```python
from build123d import *

# Parameters (mm, degrees)
PAD_DEPTH       = 5
SKETCH001_R     = 1.5
POCKET_DEPTH    = 2.751
SKETCH002_R     = 1
POCKET001_DEPTH = 5


with BuildPart() as part:
    # Sketch → Pad (new body, symmetric)
    with BuildSketch(Plane.YZ):
        with BuildLine():
            ThreePointArc((-1.299038, -0.75), (1.5, 0), (-1.299038, 0.75))
            Line((-11.299038, 0.75), (-1.299038, 0.75))
            Line((-11.299038, 2.75), (-11.299038, 0.75))
            Line((0, 2.75), (-11.299038, 2.75))
            ThreePointArc((1.2e-05, -2.75), (2.75, 6e-06), (0, 2.75))
            Line((-11.299038, -2.75), (1.2e-05, -2.75))
            Line((-11.299038, -2.75), (-11.299038, -0.75))
            Line((-11.299038, -0.75), (-1.299038, -0.75))
        make_face()
    extrude(amount=PAD_DEPTH, both=True)

    # Sketch001 → Pocket (cut, through all)
    with BuildSketch(Plane.XY):
        with Locations((0, -6)):
            Circle(SKETCH001_R)
    extrude(amount=-POCKET_DEPTH, mode=Mode.SUBTRACT)

    # Sketch002 → Pocket001 (cut)
    with BuildSketch(Plane.XY):
        with Locations((0, -6)):
            Circle(SKETCH002_R)
    extrude(amount=POCKET001_DEPTH, mode=Mode.SUBTRACT)


solid = part.part
```
The model under review builds one solid part; all positions refer to its coordinate system, in mm. A direction names the side the tool comes from. Round coordinates to 2 decimals unless told otherwise and drop trailing zeros. Loops run counter-clockwise (first coordinate to the right, second up) from the corner with the lowest first, then second, coordinate; pieces in that order, holes last.
1) Tool access review of faces 1 (the face through (-0.325, -7.464, -1.736)), 2 (the face through (-1, -7.5, -0.75)), 3 (the face through (1.2, -5.6, 2.75)): name each direction out of +Z, -Z, +X, -X, +Y, -Y from which nothing blocks a thin tool from reaching the whole face with its end or side.
Values follow:
face 1: -Z
face 2: +X, -X, -Y
face 3: +Z, +X, -X, +Y, -Y
2) Consider section D-D on x = 4.25. State the section outline as (y, z) points, then the cut area to 3 significant figures.
Values follow:
outline: (-11.3, -2.75) - (0, -2.75) arc R2.75 ccw to (0, 2.75) - (-11.3, 2.75) - (-11.3, 0.75) - (-1.3, 0.75) arc R1.5 cw (long way) to (-1.3, -0.75) - (-11.3, -0.75) - close
area: 52.2 mm2
3) Consider section B-B on y = -6. State the section outline as (x, z) points.
Values follow:
outline: (-5, -2.75) - (-1.5, -2.75) - (-1.5, -0.75) - (-5, -0.75) - close; (-5, 0.75) - (-1, 0.75) - (-1, 2.75) - (-5, 2.75) - close; (1, 0.75) - (5, 0.75) - (5, 2.75) - (1, 2.75) - close; (1.5, -2.75) - (5, -2.75) - (5, -0.75) - (1.5, -0.75) - close
4) Clearance check with a flat-ended pin moving along its axis: P1, Ø3, axis at x = -1, z = -2, coming from the +Y side. State where the tip first meets the part, or that it passes through.
Values follow:
P1: stops at y = 2.7
5) Consider section C-C on y = -1.75. State the section outline as (x, z) points, then the cut area to 3 significant figures.
Values follow:
outline: (-5, -2.75) - (5, -2.75) - (5, -0.75) - (-5, -0.75) - close; (-5, 0.75) - (5, 0.75) - (5, 2.75) - (-5, 2.75) - close
area: 40.0 mm2
6) The part is to be moulded in two halves that separate along Z. For faces 4 (the face through (0, -11.299, 2)), 5 (the face through (0.1, -7.5, 0.75)), 6 (the face through (0, -4, -2.75)), say which applies: pulls with the +Z half, pulls with the -Z half, needs draft (parallel to the pull), parting line crosses it, or undercut.
Values follow:
face 4: needs draft
face 5: undercut
face 6: pulls with the -Z half
7) Consider section A-A on x = 0. State the section outline as (y, z) points.
Values follow:
outline: (-11.3, -2.75) - (-7.5, -2.75) - (-7.5, -0.75) - (-11.3, -0.75) - close; (-11.3, 0.75) - (-7, 0.75) - (-7, 2.75) - (-11.3, 2.75) - close; (-5, 0.75) - (-1.3, 0.75) arc R1.5 cw (long way) to (-1.3, -0.75) - (-4.5, -0.75) - (-4.5, -2.75) - (0, -2.75) arc R2.75 ccw to (0, 2.75) - (-5, 2.75) - close
8) Wall thickness on line 1 along Z through (x, y) = (-4.25, -3.75); line 2 along Y through (x, z) = (-2.5, 0): over which ranges is each line inside the solid? List them lowest first.
Values follow:
line 1: z = -2.75 to -0.75, 0.75 to 2.75
line 2: y = 1.5 to 2.75
